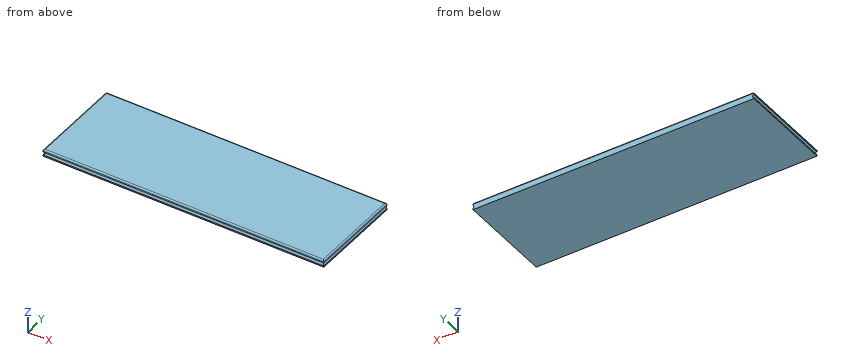
from build123d import *

# Parameters (mm, degrees)
F0_W     = 1041.4
F0_H     = 355.6
F1_DEPTH = 25.4
F2_R     = 5.08
F4_DEPTH = 355.601
F6_DEPTH = 1041.401
F8_DEPTH = 355.601


with BuildPart() as f1:
    # F0 (on Top) → F1 (new body)
    with BuildSketch(Plane.XY):
        with Locations((520.7, 177.8)):
            Rectangle(F0_W, F0_H)
    extrude(amount=-F1_DEPTH)

    # F2
    f2_edges = [f1.edges().sort_by_distance(p)[0] for p in [
        (520.7, 0, 0),
        (1041.4, 177.8, 0),
        (520.7, 355.6, 0),
        (0, 177.8, 0),
    ]]
    fillet(f2_edges, radius=F2_R)

    # F3 (on face) → F4 (cut, through all)
    with BuildSketch(Plane.XZ):
        with BuildLine():
            Line((0, -9.080117), (0, -20.479154))
            ThreePointArc((0, -20.479154), (4.683372, -14.779635), (0, -9.080117))
        make_face()
    extrude(amount=-F4_DEPTH, mode=Mode.SUBTRACT)

    # F5 (on Right) → F6 (cut, through all)
    with BuildSketch(Plane.YZ):
        with BuildLine():
            Line((0, -9.203359), (0, -20.589933))
            ThreePointArc((0, -20.589933), (3.376242, -14.896646), (0, -9.203359))
        make_face()
    extrude(amount=F6_DEPTH, mode=Mode.SUBTRACT)

    # F7 (on face) → F8 (cut, through all)
    with BuildSketch(Plane.XZ):
        with BuildLine():
            Line((1041.4, -20.478019), (1041.4, -9.203359))
            ThreePointArc((1041.4, -9.203359), (1038.527252, -14.840689), (1041.4, -20.478019))
        make_face()
    extrude(amount=-F8_DEPTH, mode=Mode.SUBTRACT)


solid = f1.part
Input: part model. Units: mm. Frame: model coordinates. Round coordinates to 2 decimals unless told otherwise and drop trailing zeros. Order: outer loops, then holes, each group sorted by start corner. A loop starts at its lowest first (then second) coordinate and runs counter-clockwise, first axis right, second up.
1. Cut plane A-A, the plane z = -14.75. Output: boundary loops of the cut face in (x, y), then the cut area to 3 significant figures.
The answers:
outline: (4.68, 3.37) - (1038.53, 3.37) - (1038.53, 355.6) - (4.68, 355.6) - close
area: 364,000 mm2
2. Material intervals for line 1 (Y direction, x = 866, z = -16.5); line 2 (X direction, y = 300.5, z = -4.75); line 3 (X direction, y = 169, z = -14), sorted ascending.
The answers:
line 1: y = 3.18 to 355.6
line 2: x = 0.01 to 1041.39
line 3: x = 4.63 to 1038.58
3. Pin query (flat end, axial travel): P1, Ø4, axis at y = 133, z = -11.5, coming from the +X side; P2, Ø8, axis at x = 654, z = -11, coming from the -Y side. Return the tip coordinate at first contact, or that it passes through.
The answers:
P1: stops at x = 1041.02
P2: stops at y = 0
